Autodesk Fusion 360 part; units mm, degrees
sphere "EsferaPrimitiva1" add diameter 13 placed x (0, 1, 0) y (0, 0, 1) z (1, 0, 0) at (0, 0, 0)
sketch "Boceto2" plane through (0, 0, 0) normal (0, 1, 0) x (1, 0, 0)
  circle A0 centre (0, 0) radius 20
  dimension "d2" = 40
sketch "Boceto1" plane through (0, 0, 0) normal (0, 1, 0) x (1, 0, 0)
  circle A0 centre (0, 0) radius 10
  line L0 (0, 0) -> (0, -13.2142)
  dimension "d1" = 20

Autodesk Fusion 360 part; units mm, degrees
sketch "Sketch1" plane through (0, 0, 0) normal (0, 0, 1) x (1, 0, 0)
  line L0 (20, -25) -> (-20, -25)
  line L1 (-20, -25) -> (-20, 25)
  line L2 (-20, 25) -> (20, 25)
  line L3 (20, 25) -> (20, -25)
  line L4 (20, -25) -> (-20, 25) construction
  line L5 (-20, -25) -> (20, 25) construction
  dimension "d1" = 40
  dimension "d2" = 50
extrude "Extrude1" add sketch "Sketch1" along normal blind 20
sketch "Sketch2" plane through (0, 25, 0) normal (0, 1, 0) x (-1, 0, 0)
  line L0 (-20, 0) -> (20, 0)
  line L1 (20, 0) -> (20, 20)
  line L2 (20, 20) -> (-20, 20)
  line L3 (-20, 20) -> (-20, 0)
  line L4 (0, 9) -> (0, 20) construction
  line L5 (0, 9) -> (0, 8) construction
  line L6 (0, 8) -> (18, 8)
  line L7 (18, 8) -> (18, 17)
  line L8 (18, 17) -> (-18, 17)
  line L9 (-18, 17) -> (-18, 8)
  line L10 (-18, 8) -> (0, 8)
  line L11 (-18, 8) -> (-18, 2) construction
  line L12 (-18, 2) -> (18, 2) construction
  line L13 (18, 2) -> (18, 8) construction
  line L14 (-18, 2) -> (18, 2)
  line L15 (18, 2) -> (18, 5)
  line L16 (18, 5) -> (-18, 5)
  line L17 (-18, 5) -> (-18, 2)
  line L18 (20, 0) -> (20, 20)
  dimension "d5" = 3
  dimension "d8" = 2
  dimension "d9" = 6
  dimension "d13" = 2
  dimension "d43" = 2
sketch "Sketch3" plane through (-20, 0, 0) normal (-1, 0, 0) x (0, -1, 0)
  line L0 (-25, 0) -> (25, 0)
  line L1 (25, 0) -> (25, 20)
  line L2 (25, 20) -> (-25, 20)
  line L3 (-25, 20) -> (-25, 0)
  line L4 (-23, 17) -> (23, 17)
  line L5 (23, 17) -> (23, 8)
  line L6 (23, 8) -> (-23, 8)
  line L7 (-23, 8) -> (-23, 17)
  line L8 (-23, 5) -> (23, 5)
  line L9 (23, 5) -> (23, 2)
  line L10 (23, 2) -> (-23, 2)
  line L11 (-23, 2) -> (-23, 5)
  dimension "d14" = 3
  dimension "d15" = 2
  dimension "d16" = 2
  dimension "d18" = 2
  dimension "d19" = 2
  dimension "d20" = 6
  dimension "d21" = 3
  dimension "d22" = 2
sketch "Sketch4" plane through (20, 0, 0) normal (1, 0, 0) x (0, 1, 0)
  line L0 (-25, 0) -> (25, 0)
  line L1 (25, 0) -> (25, 20)
  line L2 (25, 20) -> (-25, 20)
  line L3 (-25, 20) -> (-25, 0)
  line L4 (-23, 8) -> (23, 8)
  line L5 (23, 8) -> (23, 17)
  line L6 (-23, 17) -> (-23, 8)
  line L7 (23, 17) -> (-23, 17)
  line L8 (-23, 2) -> (23, 2)
  line L9 (23, 2) -> (23, 5)
  line L10 (-23, 5) -> (-23, 2)
  line L11 (23, 5) -> (-23, 5)
sketch "Sketch5" plane through (0, -25, 0) normal (0, -1, 0) x (1, 0, 0)
  line L0 (-20, 0) -> (20, 0)
  line L1 (20, 0) -> (20, 20)
  line L2 (20, 20) -> (-20, 20)
  line L3 (-20, 20) -> (-20, 0)
  line L4 (-18, 8) -> (-18, 17)
  line L5 (-18, 17) -> (18, 17)
  line L6 (18, 17) -> (18, 8)
  line L7 (0, 8) -> (-18, 8)
  line L8 (18, 8) -> (0, 8)
  line L9 (18, 2) -> (-18, 2)
  line L10 (-18, 2) -> (-18, 5)
  line L11 (18, 5) -> (18, 2)
  line L12 (-18, 5) -> (18, 5)
extrude "Extrude2" cut sketch "Sketch2" against normal blind 1.5 contours L6 L7 L8 L9 L10 | L14 L15 L16 L17
extrude "Extrude3" cut sketch "Sketch3" against normal blind 1.5 contours L4 L5 L6 L7 | L8 L9 L10 L11
extrude "Extrude4" cut sketch "Sketch5" against normal blind 1.5 contours L4 L5 L6 L7 L8 | L9 L10 L11 L12
extrude "Extrude5" cut sketch "Sketch4" against normal blind 1.5 contours L4 L5 L6 L7 | L8 L9 L10 L11
chamfer "Chamfer1" distance 1.5 angle 45 5 edges at (18, 23.5, 12.5) (0, 23.5, 17) (-18, 23.5, 12.5) (0, 23.5, 8) (18.5, 0, 8) 3 faces at (18.5, -7.6667, 14) (-6, -23.5, 14) (-18.5, 7.6667, 14)
sketch "Sketch6" plane through (0, 0, 20) normal (0, 0, 1) x (-1, 0, 0)
  line L0 (-20, -25) -> (20, -25)
  line L1 (20, -25) -> (20, 25)
  line L2 (20, 25) -> (-20, 25)
  line L3 (-20, 25) -> (-20, -25)
  line L4 (-17.5, 22.5) -> (17.5, 22.5)
  line L5 (17.5, 22.5) -> (17.5, -22.5)
  line L6 (17.5, -22.5) -> (-17.5, -22.5)
  line L7 (-17.5, -22.5) -> (-17.5, 22.5)
  line L8 (-17.5, 22.5) -> (17.5, -22.5) construction
  line L9 (17.5, 22.5) -> (-17.5, -22.5) construction
  dimension "d29" = 2.5
  dimension "d30" = 2.5
extrude "Extrude6" cut sketch "Sketch6" against normal blind 18 contours L4 L5 L6 L7
sketch "Sketch7" plane through (0, -25, 0) normal (0, -1, 0) x (1, 0, 0)
  line L0 (18, 2) -> (-18, 2)
  line L1 (-18, 5) -> (18, 5)
  line L2 (18, 5) -> (18, 2)
  line L3 (-20, 0) -> (20, 0)
  line L4 (20, 0) -> (20, 20)
  line L5 (20, 20) -> (-20, 20)
  line L6 (-20, 20) -> (-20, 0)
  line L7 (0, 0) -> (0, 20)
  line L8 (0, 0) -> (-5, 0) construction
  line L9 (-5, 0) -> (-5, 6)
  line L10 (-5, 6) -> (-10, 6)
  line L11 (-10, 6) -> (-15, 0)
  line L12 (-5, 0) -> (-15, 0)
  line L13 (10, 6) -> (15, 0)
  line L14 (5, 0) -> (15, 0)
  line L15 (5, 6) -> (10, 6)
  line L16 (5, 0) -> (5, 6)
  line L17 (-18, 17) -> (18, 17)
  line L18 (18, 17) -> (18, 8)
  line L19 (18, 8) -> (-18, 8)
  line L20 (-18, 8) -> (-18, 17)
  line L21 (-18, 2) -> (-18, 5)
  dimension "d33" = 6
  dimension "d34" = 5
  dimension "d35" = 10
  dimension "d36" = 5
extrude "Extrude7" add sketch "Sketch7" along normal blind 0.8 and the other way blind 2 contours L0 L3 L13 L14 L16 | L0 L1 L13 L16 | L1 L13 L15 L16 | L0 L3 L9 L11 L12 | L0 L1 L9 L11 | L1 L9 L10 L11
mirror "Mirror1" about plane through (0, 0, 0) normal (0, 1, 0) of "Extrude7"
The model under review builds one solid part; all positions refer to its coordinate system, in mm. A direction names the side the tool comes from. Coordinates: 2 decimals unless noted, no trailing zeros. Answer in a Markdown table with one row per item. Add a question column.
Item 1: Clearance check with flat-ended pins moving along their axes: pin 1 (1.5 mm diameter, centred on x = 15, z = 4, fed in from -Y); pin 2 (1.2 mm diameter, centred on x = -19.5, z = 4, fed in from +Y); pin 3 (3 mm diameter, centred on x = -9.5, y = 3, fed in from -Z). State where each tip first meets the part, or that it passes through.
Item 2: Mouldability with a two-part tool opening along Z and no side actions: class faces 1 (the flat face through (14, -24, 5)), 2 (the flat face through (-17.5, 0, 11)) as +Z half, -Z half, draft (parallel to the pull), parting line (faces both ways), or undercut.
Item 3: To check wall thickness, follow probe 1 along Y at (x, z) = (-2.5, 14.5); probe 2 along X at (y, z) = (-11, 4.5); probe 3 along X at (y, z) = (9.5, 19.25). State the ranges of each line that lie inside material, in increasing order.
Item 4: Machinability: for faces 3 (the flat face through (0, -24, 9)), 4 (the flat face through (12, 24.9, 3.6)), 5 (the flat face through (19, 0, 2)), which of the approach directions +Z, -Z, +X, -X, +Y, -Y give a long, thin tool a straight path to every point of the face, cutting with its end or side? Answer none if there is none.
Final values:
| question | item | result |
|---|---|---|
| 1 | pin 1 | stops at y = -23.5 |
| 1 | pin 2 | stops at y = 25 |
| 1 | pin 3 | stops at z = 0 |
| 2 | face 1 | undercut |
| 2 | face 2 | draft |
| 3 | probe 1 | y = -23.5 to -22.5, 22.5 to 23.5 |
| 3 | probe 2 | x = -18.5 to -17.5, 17.5 to 18.5 |
| 3 | probe 3 | x = -20 to -17.5, 17.5 to 20 |
| 4 | face 3 | -Y |
| 4 | face 4 | +Y |
| 4 | face 5 | +X |
